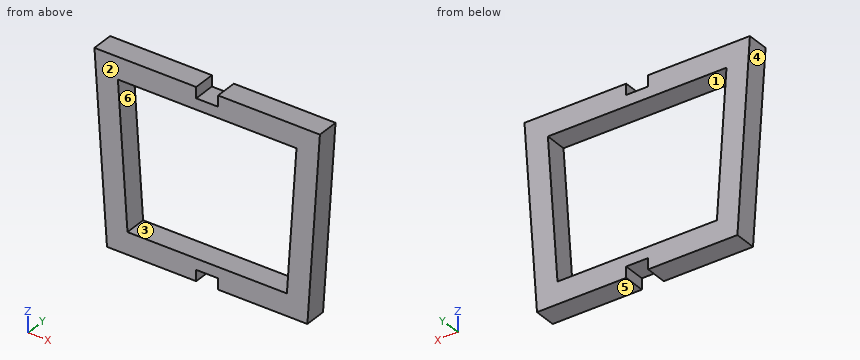
from build123d import *

# Parameters (mm, degrees)
F2_DEPTH = 17.5
F3_DEPTH = 17.5
F4_W     = 35
F4_H     = 17.5
F5_DEPTH = 35
F6_W     = 35
F6_H     = 17.5
F7_DEPTH = 35


with BuildPart() as f2:
    # F0 (on Front) → F2 (new body, symmetric)
    with BuildSketch(Plane.XZ):
        Polygon((180, 150), (-180, 150), (-160, -150), (160, -150), align=None)
    extrude(amount=F2_DEPTH, both=True)

    # F1 (on face) → F3 (cut, symmetric)
    with BuildSketch(Plane.XZ):
        Polygon((142.588975, 115), (-142.588975, 115), (-127.255642, -115), (127.255642, -115), align=None)
    extrude(amount=F3_DEPTH, both=True, mode=Mode.SUBTRACT)

    # F4 (on face) → F5 (cut)
    with BuildSketch(Plane.XZ.offset(17.5)):
        with Locations((0, -141.25)):
            Rectangle(F4_W, F4_H)
    extrude(amount=-F5_DEPTH, mode=Mode.SUBTRACT)

    # F6 (on face) → F7 (cut)
    with BuildSketch(Plane.XZ.offset(17.5)):
        with Locations((0, 141.25)):
            Rectangle(F6_W, F6_H)
    extrude(amount=-F7_DEPTH, mode=Mode.SUBTRACT)


solid = f2.part
Verification items for the finished model (mm, model axes). Face numbers are marked on the shaded views. A direction names the side the tool comes from. Round coordinates to 2 decimals unless told otherwise and drop trailing zeros. Order: outer loops, then holes, each group sorted by start corner. A loop starts at its lowest first (then second) coordinate and runs counter-clockwise, first axis right, second up.
1. Section check C-C on x = -106. Record the cut outline in (y, z), then the cut area to 3 significant figures.
Final values:
outline: (-17.5, -150) - (17.5, -150) - (17.5, -115) - (-17.5, -115) - close; (-17.5, 115) - (17.5, 115) - (17.5, 150) - (-17.5, 150) - close
area: 2,450 mm2
2. Thickness scan on L1, parallel to Z at x = -81.5, y = -15; L2, parallel to Z at x = -1.5, y = 16; L3, parallel to X at y = 8.5, z = -113. Record the ranges inside material, lowest first.
Final values:
L1: z = -150 to -115, 115 to 150
L2: z = -132.5 to -115, 115 to 132.5
L3: x = -162.47 to -127.39, 127.39 to 162.47
3. Go/stop test with flat-tipped pins: P1, Ø12, axis at y = -13, z = 100, coming from the +X side; P2, Ø12, axis at y = 1.5, z = -60, coming from the +X side; P3, Ø17.5, axis at x = 4.5, y = -7, coming from the +Z side. Record where each tip stops, or that it passes through.
Final values:
P1: stops at x = 177.07
P2: stops at x = 166.4
P3: stops at z = 132.5
4. Release check for a two-part mould opening along X. For the marked faces 1, 2, 3 and 4 record: +X half, -X half, draft (parallel to the pull), parting line (faces both ways), or undercut.
Final values:
face 1: undercut
face 2: draft
face 3: undercut
face 4: -X half
5. Access from +Z, -Z, +X, -X, +Y, -Y to the whole of each face (thin tool, end or side, straight path). Record for the marked faces 5 and 6.
Final values:
face 5: -Z, +X, -X, +Y, -Y
face 6: +Y, -Y
6. Section check D-D on z = -128. Record the cut outline in (x, y), then the cut area to 3 significant figures.
Final values:
outline: (-161.47, -17.5) - (161.47, -17.5) - (161.47, 17.5) - (-161.47, 17.5) - close
area: 11,300 mm2
7. Section check B-B on y = -1. Record the cut outline in (x, z), then the cut area to 3 significant figures.
Final values:
outline: (-180, 150) - (-160, -150) - (-17.5, -150) - (-17.5, -132.5) - (17.5, -132.5) - (17.5, -150) - (160, -150) - (180, 150) - (17.5, 150) - (17.5, 132.5) - (-17.5, 132.5) - (-17.5, 150) - close; hole (-142.59, 115) - (-127.26, -115) - (127.26, -115) - (142.59, 115) - close
area: 38,700 mm2
8. Section check A-A on x = 10. Record the cut outline in (y, z).
Final values:
outline: (-17.5, -132.5) - (17.5, -132.5) - (17.5, -115) - (-17.5, -115) - close; (-17.5, 115) - (17.5, 115) - (17.5, 132.5) - (-17.5, 132.5) - close
